```python
from build123d import *

# Parameters (mm, degrees)
ESBO_O1_R                = 5.05
RESSALTO_EXTRUS_O2_DEPTH = 1.8
ESBO_O2_W                = 49.1
ESBO_O2_H                = 29.842997711
ESBO_O2_R                = 5.05
RESSALTO_EXTRUS_O3_DEPTH = 1.8
RESSALTO_EXTRUS_O5_START = 1.5
ESBO_O3_R                = 4.05
RESSALTO_EXTRUS_O5_DEPTH = 1.5


with BuildPart() as part:
    # Esboço1 → Ressalto-extrusão2 (new body)
    with BuildSketch(Plane.XY):
        with BuildLine():
            Line((9.899494937, 9.899494937), (-14.345555324, 34.144545197))
            Line((-14.345555324, 34.144545197), (-55.882327004, 34.144545197))
            Line((-55.882327004, 34.144545197), (-55.882327004, 4.301547486))
            Line((-55.882327004, 4.301547486), (-24.020751859, 4.301547486))
            Line((-24.020751859, 4.301547486), (-8.97177071, -10.747433663))
            ThreePointArc((-8.97177071, -10.747433663), (10.333880356, -9.445153085), (9.899494937, 9.899494937))
        make_face()
        Circle(ESBO_O1_R, mode=Mode.SUBTRACT)
    extrude(amount=RESSALTO_EXTRUS_O2_DEPTH)

    # Esboço2 → Ressalto-extrusão3 (add)
    with BuildSketch(Plane(origin=(-55.882327004, 0, 0), x_dir=(0, 0, -1), z_dir=(1, 0, 0))):
        with Locations((24.55, 19.223046342)):
            Rectangle(ESBO_O2_W, ESBO_O2_H)
        with Locations((22.7, 19.213463732)):
            Circle(ESBO_O2_R, mode=Mode.SUBTRACT)
    extrude(amount=RESSALTO_EXTRUS_O3_DEPTH)

    # Esboço3 → Ressalto-extrusão5 (add)
    with BuildSketch(Plane(origin=(0, 0, -49.1), x_dir=(-1, 0, 0), z_dir=(0, 0, -1)).offset(RESSALTO_EXTRUS_O5_START)):
        with BuildLine():
            Line((-9.899494937, 9.899494937), (14.345555324, 34.144545197))
            Line((14.345555324, 34.144545197), (55.882327004, 34.144545197))
            Line((55.882327004, 34.144545197), (55.882327004, 4.301547486))
            Line((55.882327004, 4.301547486), (24.020751859, 4.301547486))
            Line((24.020751859, 4.301547486), (9.899494937, -9.899494937))
            ThreePointArc((9.899494937, -9.899494937), (-9.899494937, -9.899494937), (-9.899494937, 9.899494937))
        make_face()
        Circle(ESBO_O3_R, mode=Mode.SUBTRACT)
    extrude(amount=-RESSALTO_EXTRUS_O5_DEPTH)


solid = part.part
```
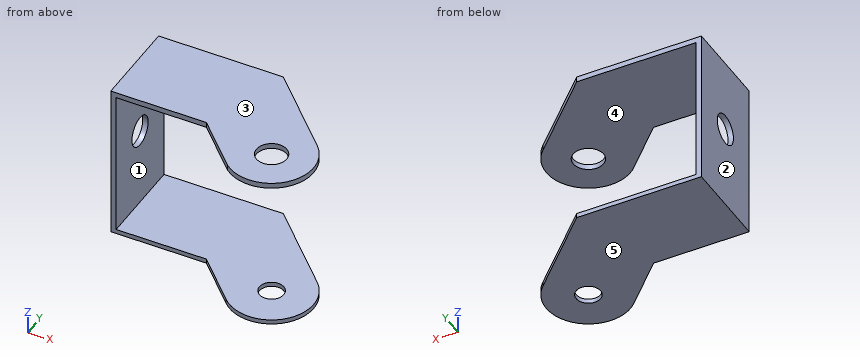
Check sheet for the modelled part. Datum: model origin and axes. Units: mm. Face numbers are marked on the shaded views. A direction names the side the tool comes from. Give positions to 0.01 mm unless a question says otherwise; leave off trailing zeros. Order: outer loops, then holes, each group sorted by start corner. A loop starts at its lowest first (then second) coordinate and runs counter-clockwise, first axis right, second up. Notation, with made-up numbers: M 74.5,84.25 L 94.5,84.25 A15 ccw 94.5,105.25 Z; hole C 71,14 d11. An arc over 180 degrees is marked long. Answer in a Markdown table with one row per item. Add a question column.
Q1. Sectioned sample at A-A, the plane x = -37. Record the boundary of the cut face in (y, z).
Q2. Release check for a two-part mould opening along Z. For the marked faces 3, 4 and 5 record: released by +Z, released by -Z, zero draft, split by the parting line, or undercut.
Q3. Gauge pin test, flat ends, axial feed: pin 1 Ø11.5 at (y, z) = (19.21, -22.7) entering from -X; pin 2 Ø8 at (x, y) = (0, 0) entering from -Z; pin 3 Ø9 at (y, z) = (14, -21.5) entering from +X. Record the tip position at first contact, or that the pin passes through.
Q4. Access from +Z, -Z, +X, -X, +Y, -Y to the whole of each face (thin tool, end or side, straight path). Record for the marked faces 1 and 2.
Q5. Sectioned sample at D-D, the plane y = 0. Record the boundary of the cut face in (x, z), and give its area (3 significant figures).
Q6. Sectioned sample at B-B, the plane z = -22.7. Record the boundary of the cut face in (x, y), and give its area (3 significant figures).
Q7. Sectioned sample at C-C, the plane x = 0. Record the boundary of the cut face in (y, z), and give its area (3 significant figures).
Q8. Thickness scan on L1, parallel to Z at x = -17.5, y = 15; L2, parallel to X at y = 14, z = -45.5; L3, parallel to Y at x = 0, z = 0.7. Record the ranges inside material, lowest first.
Verdict:
| question | item | result |
|---|---|---|
| 1 | outline | M 4.3,-50.6 L 34.14,-50.6 L 34.14,-49.1 L 4.3,-49.1 Z; M 4.3,0 L 34.14,0 L 34.14,1.8 L 4.3,1.8 Z |
| 2 | face 3 | released by +Z |
| 2 | face 4 | undercut |
| 2 | face 5 | released by -Z |
| 3 | pin 1 | x = -55.88 |
| 3 | pin 2 | through |
| 3 | pin 3 | x = -54.08 |
| 4 | face 1 | +X, +Y, -Y |
| 4 | face 2 | +Z, -Z, -X, +Y, -Y |
| 5 | outline | M -19.74,-50.6 L -4.05,-50.6 L -4.05,-49.1 L -19.74,-49.1 Z; M -19.72,0 L -5.05,0 L -5.05,1.8 L -19.72,1.8 Z; M 4.05,-50.6 L 14,-50.6 L 14,-49.1 L 4.05,-49.1 Z; M 5.05,0 L 14,0 L 14,1.8 L 5.05,1.8 Z |
| 5 | area | 81.0 mm² |
| 6 | outline | M -55.88,4.3 L -54.08,4.3 L -54.08,14.16 L -55.88,14.16 Z; M -55.88,24.26 L -54.08,24.26 L -54.08,34.14 L -55.88,34.14 Z |
| 6 | area | 35.5 mm² |
| 7 | outline | M -14,-50.6 L -4.05,-50.6 L -4.05,-49.1 L -14,-49.1 Z; M -14,0 L -5.05,0 L -5.05,1.8 L -14,1.8 Z; M 4.05,-50.6 L 19.8,-50.6 L 19.8,-49.1 L 4.05,-49.1 Z; M 5.05,0 L 19.8,0 L 19.8,1.8 L 5.05,1.8 Z |
| 7 | area | 81.2 mm² |
| 8 | L1 | -50.6 to -49.1, 0 to 1.8 |
| 8 | L2 | -55.88 to -54.08 |
| 8 | L3 | -14 to -5.05, 5.05 to 19.8 |
